```python
from build123d import *

# Parameters (mm, degrees)
SKETCH1_R           = 4.7625
BOSS_EXTRUDE1_DEPTH = 25.4
SKETCH2_R           = 3.175
CUT_EXTRUDE1_DEPTH  = 32.115
SKETCH3_W           = 12.7
SKETCH3_H           = 28.80549591
CUT_EXTRUDE2_DEPTH  = 93.075


with BuildPart() as part:
    # Sketch1 → Boss-Extrude1 (new body)
    with BuildSketch(Plane.XY):
        with BuildLine():
            Line((50.8, 15.875), (0, 15.875))
            ThreePointArc((0, 15.875), (-3.361595996, 15.262087149), (-6.29056934, 13.502227791))
            Line((-6.29056934, 13.502227791), (-31.75, -8.89))
            Line((-31.75, -8.89), (-31.75, -15.24))
            Line((-31.75, -15.24), (40.675165573, -15.24))
            Line((40.675165573, -15.24), (57.09056934, -0.802227791))
            ThreePointArc((57.09056934, -0.802227791), (59.712087149, 9.711595996), (50.8, 15.875))
        make_face()
        with Locations((0, 6.35)):
            Circle(SKETCH1_R, mode=Mode.SUBTRACT)
        with Locations((50.8, 6.35)):
            Circle(SKETCH1_R, mode=Mode.SUBTRACT)
    extrude(amount=BOSS_EXTRUDE1_DEPTH)

    # Sketch2 → Cut-Extrude1 (cut, through all)
    with BuildSketch(Plane(origin=(0, -15.24, 0), x_dir=(-1, 0, 0), z_dir=(0, -1, 0))):
        with Locations((-19.05, -12.7)):
            Circle(SKETCH2_R)
        with Locations((19.05, -12.7)):
            Circle(SKETCH2_R)
    extrude(amount=-CUT_EXTRUDE1_DEPTH, mode=Mode.SUBTRACT)

    # Sketch3 → Cut-Extrude2 (cut, through all)
    with BuildSketch(Plane.ZY.offset(31.75)):
        with Locations((12.7, 5.512747955)):
            Rectangle(SKETCH3_W, SKETCH3_H)
    extrude(amount=-CUT_EXTRUDE2_DEPTH, mode=Mode.SUBTRACT)


solid = part.part
```
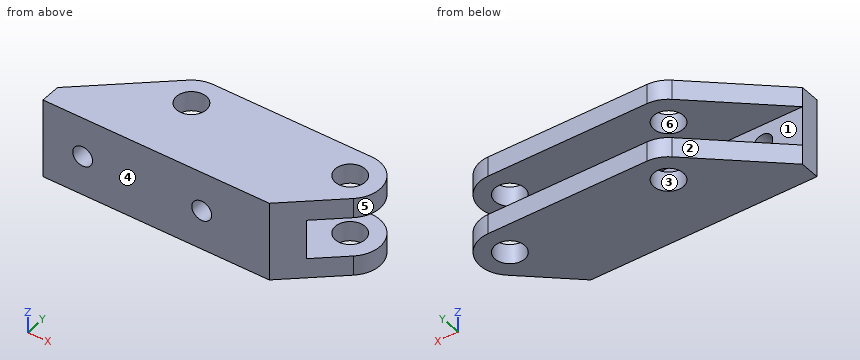
For this review, take the finished solid that the model builds, in its own axes (mm). Face numbers are marked on the shaded views. A direction names the side the tool comes from. Round coordinates to 2 decimals unless told otherwise and drop trailing zeros. Write each loop counter-clockwise with the first axis right and the second up, starting at its lowest first coordinate (ties: lowest second). Pieces come first, ordered by that corner, then holes. Notation, with made-up numbers: (21.5, 24.5) -> (76.5, 24.5) arc R31 cw to (76.5, 53.5) -> close; hole circle Ø3 at (37, -40). An arc over 180 degrees is marked (long way). One line per question, with ' | ' between items. Start each with the question number.
(1) Add section D-D, the plane x = 6.5. Write out the cut boundary in (y, z) (3 decimals).
(2) Insertion check: P1, Ø10, axis at x = -19.05, z = 12.7, coming from the +Y side; P2, Ø2, axis at x = 2.5, y = 8.5, coming from the +Z side; P3, Ø8, axis at y = -3, z = 17, coming from the +X side. Each pin has a flat end and moves straight along its axis. Give the tip position at first contact, or say it passes through.
(3) Add section C-C, the plane y = 6.35. Give the number of separate pieces and of enclosed holes in the cut face, plus the area to 3 significant figures.
(4) Add section B-B, the plane x = 19.05. Write out the cut boundary in (y, z) (3 decimals), plus the area to 3 significant figures.
(5) For line 1 along Y through (x, z) = (0, 4.75) (1 decimal); line 2 along X through (y, z) = (6.35, 24) (1 decimal); line 3 along Z through (x, y) = (23, 15.5), list the stretches that pass through material, from the lowest coordinate up. Write a range as from..to.
(6) Mouldability with a two-part tool opening along X and no side actions: class the marked faces 3, 4, 5 and 6 as released by +X, released by -X, zero draft, split by the parting line, or undercut.
(7) Tool access review of the marked faces 1 and 2: name each direction out of +Z, -Z, +X, -X, +Y, -Y from which nothing blocks a thin tool from reaching the whole face with its end or side.
(8) Add section A-A, the plane z = 12.7. Write out the cut boundary in (x, y) (3 decimals).
Answer list:
1) outline: (-15.24, 0) -> (15.875, 0) -> (15.875, 6.35) -> (-8.89, 6.35) -> (-8.89, 19.05) -> (15.875, 19.05) -> (15.875, 25.4) -> (-15.24, 25.4) -> close
2) P1: y = -8.89 | P2: through | P3: x = 58.27
3) separate pieces: 6 | enclosed holes: 0 | area: 707 mm²
4) outline: (-15.24, 0) -> (15.875, 0) -> (15.875, 6.35) -> (-8.89, 6.35) -> (-8.89, 9.525) -> (-15.24, 9.525) -> close; (-15.24, 15.875) -> (-8.89, 15.875) -> (-8.89, 19.05) -> (15.875, 19.05) -> (15.875, 25.4) -> (-15.24, 25.4) -> close | area: 435 mm²
5) line 1: -15.2..1.6, 11.1..15.9 | line 2: -14.4..-4.8, 4.8..46, 55.6..60.3 | line 3: 0..6.35, 19.05..25.4
6) face 3: undercut | face 4: zero draft | face 5: released by +X | face 6: undercut
7) face 1: +X, -X, +Y | face 2: +Z, -Z, -X, +Y
8) outline: (-31.75, -15.24) -> (-22.225, -15.24) -> (-22.225, -8.89) -> (-31.75, -8.89) -> close; (-15.875, -15.24) -> (15.875, -15.24) -> (15.875, -8.89) -> (-15.875, -8.89) -> close; (22.225, -15.24) -> (40.675, -15.24) -> (47.895, -8.89) -> (22.225, -8.89) -> close
